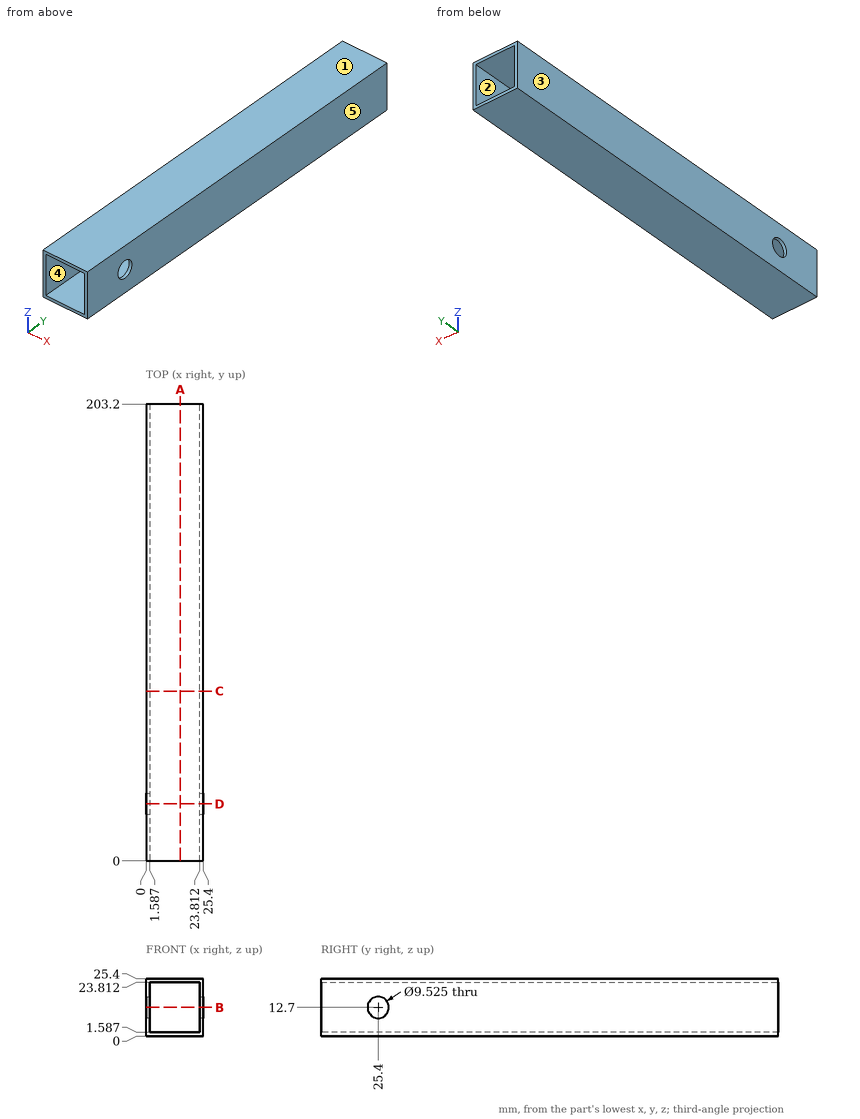
Source: three-view drawing plus pictorial views. Frame: mm from the lowest corner of the part. A direction names the side the tool comes from. Round coordinates to 2 decimals unless told otherwise and drop trailing zeros. Write each loop counter-clockwise with the first axis right and the second up, starting at its lowest first coordinate (ties: lowest second). Pieces come first, ordered by that corner, then holes. Notation, with made-up numbers: M -25.75,36 L 7.25,36 A19 ccw 7.25,47 Z; hole C 48.5,84.5 d8. An arc over 180 degrees is marked long. Write each question's results on one line, items separated by ' | '.
Q1. Access query for the marked faces 4 and 5. Directions: +Z, -Z, +X, -X, +Y, -Y. A direction counts if a zero-diameter tool reaches every point of the face in a straight line with its end or side. Return the directions, or none.
Results:
face 4: +Y, -Y | face 5: +Z, -Z, +X, +Y, -Y
Q2. Section query C-C (y = 75.5). Return loops of the section in (x, z).
Results:
outline: M 0,0 L 25.4,0 L 25.4,25.4 L 0,25.4 Z; hole M 1.59,1.59 L 23.81,1.59 L 23.81,23.81 L 1.59,23.81 Z
Q3. Section query B-B (z = 12.7). Return loops of the section in (x, y).
Results:
outline: M 0,0 L 1.59,0 L 1.59,20.64 L 0,20.64 Z; M 0,30.16 L 1.59,30.16 L 1.59,203.2 L 0,203.2 Z; M 23.81,0 L 25.4,0 L 25.4,20.64 L 23.81,20.64 Z; M 23.81,30.16 L 25.4,30.16 L 25.4,203.2 L 23.81,203.2 Z
Q4. Draft query along Z for the marked faces 1, 2 and 3. Return one class per face: released by +Z, released by -Z, zero draft, split by the parting line, or undercut.
Results:
face 1: released by +Z | face 2: undercut | face 3: zero draft
Q5. Section query D-D (y = 25.4). Return loops of the section in (x, z).
Results:
outline: M 0,0 L 25.4,0 L 25.4,7.94 L 23.81,7.94 L 23.81,1.59 L 1.59,1.59 L 1.59,7.94 L 0,7.94 Z; M 0,17.46 L 1.59,17.46 L 1.59,23.81 L 23.81,23.81 L 23.81,17.46 L 25.4,17.46 L 25.4,25.4 L 0,25.4 Z
Q6. Section query A-A (x = 15.25). Return loops of the section in (y, z).
Results:
outline: M 0,0 L 203.2,0 L 203.2,1.59 L 0,1.59 Z; M 0,23.81 L 203.2,23.81 L 203.2,25.4 L 0,25.4 Z
Q7. Line query: line 1 along Z through (x, y) = (15, 140); line 2 along Y through (x, z) = (25, 12.7). Output: solid intervals per line, ascending.
Results:
line 1: z = 0 to 1.59, 23.81 to 25.4 | line 2: y = 0 to 20.64, 30.16 to 203.2
Q8. Pin query (flat end, axial travel): P1, Ø8, axis at x = 13, y = 151.5, coming from the -Z side. Return the tip coordinate at first contact, or that it passes through.
Results:
P1: stops at z = 0
